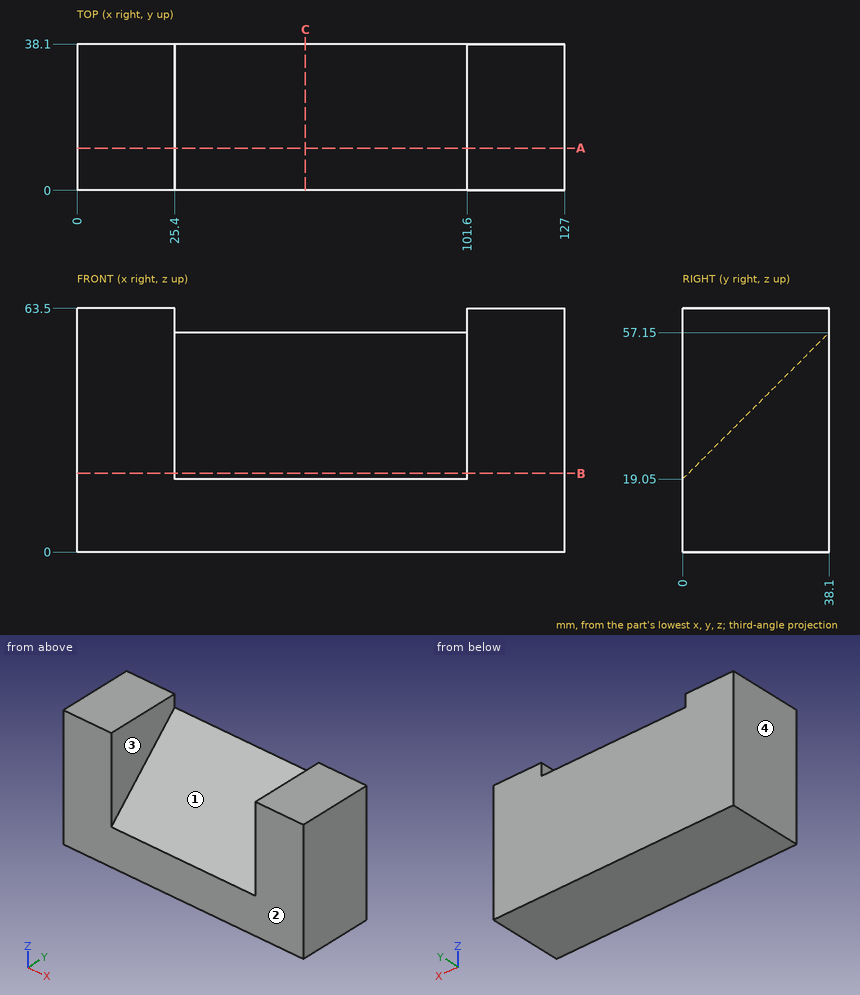
Input: dimensioned drawing with shaded views. Units: mm. Origin: part minimum x, y, z. Give positions to 0.01 mm unless a question says otherwise; leave off trailing zeros. Write each loop counter-clockwise with the first axis right and the second up, starting at its lowest first coordinate (ties: lowest second). Pieces come first, ordered by that corner, then holes.
Q1. Material intervals for probe 1 along X at (y, z) = (2.5, 50); probe 2 along Z at (x, y) = (59.5, 26); probe 3 along Z at (x, y) = (54.5, 4), sorted ascending.
Q2. Section B-B, the plane z = 20.5. Output: boundary loops of the cut face in (x, y).
Q3. Section C-C, the plane x = 59.5. Output: boundary loops of the cut face in (y, z), plus the area to 3 significant figures.
Q4. Pull-direction query (X, two-part tool) for the marked faces 1, 2, 3 and 4; classes: pulls with the +X half, pulls with the -X half, needs draft (parallel to the pull), parting line crosses it, or undercut.
Q5. Section A-A, the plane y = 11. Output: boundary loops of the cut face in (x, z).
Q6. First-contact query: P1, Ø12, axis at x = 47, z = 39.5, coming from the -Y side; P2, Ø4, axis at x = 46.5, z = 53, coming from the -Y side; P3, Ø5, axis at x = 36, y = 32, coming from the +Z side. Flat tips, straight axial feed; report the tip coordinate or a pass-through.
Filled in:
1. probe 1: x = 0 to 25.4, 101.6 to 127
1. probe 2: z = 0 to 45.05
1. probe 3: z = 0 to 23.05
2. outline: (0, 0) - (25.4, 0) - (25.4, 1.45) - (101.6, 1.45) - (101.6, 0) - (127, 0) - (127, 38.1) - (0, 38.1) - close
3. outline: (0, 0) - (38.1, 0) - (38.1, 57.15) - (0, 19.05) - close
3. area: 1,450 mm2
4. face 1: undercut
4. face 2: needs draft
4. face 3: undercut
4. face 4: pulls with the -X half
5. outline: (0, 0) - (127, 0) - (127, 63.5) - (101.6, 63.5) - (101.6, 30.05) - (25.4, 30.05) - (25.4, 63.5) - (0, 63.5) - close
6. P1: stops at y = 14.45
6. P2: stops at y = 31.95
6. P3: stops at z = 53.55
